from build123d import *

# Parameters (mm, degrees)
SKETCH1_W           = 200
SKETCH1_H           = 120
BOSS_EXTRUDE3_DEPTH = 10
SKETCH3_R           = 5
SKETCH3_W           = 160
SKETCH3_H           = 80
CUT_EXTRUDE2_DEPTH  = 5
SKETCH6_R           = 9
SKETCH6_R_2         = 5.25
BOSS_EXTRUDE4_DEPTH = 10
CHAMFER1_SIZE       = 1


with BuildPart() as part:
    # Sketch1 → Boss-Extrude3 (new body)
    with BuildSketch(Plane(origin=(0, 0, 0), x_dir=(1, 0, 0), z_dir=(0, 1, 0))):
        Rectangle(SKETCH1_W, SKETCH1_H)
    extrude(amount=BOSS_EXTRUDE3_DEPTH)

    # Sketch3 → Cut-Extrude2 (cut)
    with BuildSketch(Plane(origin=(0, 10, 0), x_dir=(1, 0, 0), z_dir=(0, 1, 0))):
        with Locations(Location((-90, 50, 0), (0, 0, 270))):
            Circle(SKETCH3_R)
        with Locations(Location((90, -50, 0), (0, 0, 270))):
            Circle(SKETCH3_R)
        with Locations(Location((90, 50, 0), (0, 0, 270))):
            Circle(SKETCH3_R)
        with Locations(Location((-90, -50, 0), (0, 0, 270))):
            Circle(SKETCH3_R)
        Rectangle(SKETCH3_W, SKETCH3_H)
    extrude(amount=-CUT_EXTRUDE2_DEPTH, mode=Mode.SUBTRACT)

    # Sketch6 → Boss-Extrude4 (add)
    # profile 1 of 4: a face of its own
    with BuildSketch(Plane(origin=(0, 5, 0), x_dir=(1, 0, 0), z_dir=(0, 1, 0))):
        with Locations(Location((-90, 50, 0), (0, 0, 270))):
            Circle(SKETCH6_R)
        with Locations(Location((-90, 50, 0), (0, 0, 270))):
            Circle(SKETCH6_R_2, mode=Mode.SUBTRACT)
    # profile 2 of 4: a face of its own
    with BuildSketch(Plane(origin=(0, 5, 0), x_dir=(1, 0, 0), z_dir=(0, 1, 0))):
        with Locations(Location((90, 50, 0), (0, 0, 270))):
            Circle(SKETCH6_R)
        with Locations(Location((90, 50, 0), (0, 0, 270))):
            Circle(SKETCH6_R_2, mode=Mode.SUBTRACT)
    # profile 3 of 4: a face of its own
    with BuildSketch(Plane(origin=(0, 5, 0), x_dir=(1, 0, 0), z_dir=(0, 1, 0))):
        with Locations(Location((90, -50, 0), (0, 0, 270))):
            Circle(SKETCH6_R)
        with Locations(Location((90, -50, 0), (0, 0, 270))):
            Circle(SKETCH6_R_2, mode=Mode.SUBTRACT)
    # profile 4 of 4: a face of its own
    with BuildSketch(Plane(origin=(0, 5, 0), x_dir=(1, 0, 0), z_dir=(0, 1, 0))):
        with Locations(Location((-90, -50, 0), (0, 0, 270))):
            Circle(SKETCH6_R)
        with Locations(Location((-90, -50, 0), (0, 0, 270))):
            Circle(SKETCH6_R_2, mode=Mode.SUBTRACT)
    extrude(amount=BOSS_EXTRUDE4_DEPTH)

    # Chamfer1
    chamfer1_edges = [part.edges().sort_by_distance(p)[0] for p in [
        (-90, 10, -59),
        (90, 10, -59),
        (90, 10, 41),
        (-90, 10, 41),
    ]]
    chamfer(chamfer1_edges, length=CHAMFER1_SIZE - 0.0001)  # a hair under: the kernel refuses the full size


solid = part.part
Work out the finished part from the listing and answer in its coordinate system (mm). A direction names the side the tool comes from. Coordinates: 2 decimals unless noted, no trailing zeros. Write each loop counter-clockwise with the first axis right and the second up, starting at its lowest first coordinate (ties: lowest second). Pieces come first, ordered by that corner, then holes. Notation, with made-up numbers: M -13,64 L 14,64 A26 ccw 14,96 Z; hole C 82,59.25 d11. An arc over 180 degrees is marked long. Answer as CSV lines item,"result". Start each with the question number.
Item 1: Consider L1, parallel to X at y = 12.4, z = -50; L2, parallel to X at y = 7.75, z = 15; L3, parallel to Z at x = 35.5, y = 6. Determine where each line is inside the solid, lowest interval first.
Item 2: A tool of negligible diameter and unlimited length cuts with its end or side. For faces 1 (the face through (-1, 0, -1)), 2 (the face through (-1, 10, -41)), from which of +Z, -Z, +X, -X, +Y, -Y can it reach the whole face along a straight path? Write none if from no direction.
Item 3: Section A-A on x = -48.5 is taken. Write down the section's boundary in (y, z).
Item 4: Section C-C on z = -10.5 is taken. Write down the section's boundary in (x, y).
Item 5: Determine the mould class of faces 3 (the face through (-94.88, 7.54, 48.92)), 4 (the face through (86, 15, 54)), 5 (the face through (-1, 5, -1)), 6 (the face through (-1, 5, -60)) for opening direction Z: released by +Z, released by -Z, zero draft, split by the parting line, or undercut.
Item 6: A flat-ended cylindrical pin translates along its axis: P1, Ø4, axis at x = -50, z = 11.5, coming from the +Y side. Find the tip coordinate at first contact, or state that the pin passes through.
Checks:
1,L1,"x = -99 to -95.25, -84.75 to -81, 81 to 84.75, 95.25 to 99"
1,L2,"x = -100 to -80, 80 to 100"
1,L3,"z = -60 to -40, 40 to 60"
2,face 1,"+Z, -Z, +X, -X, -Y"
2,face 2,"+Y"
3,outline,"M 0,-60 L 10,-60 L 10,-40 L 5,-40 L 5,40 L 10,40 L 10,60 L 0,60 Z"
4,outline,"M -100,0 L 100,0 L 100,10 L 80,10 L 80,5 L -80,5 L -80,10 L -100,10 Z"
5,face 3,"undercut"
5,face 4,"zero draft"
5,face 5,"undercut"
5,face 6,"released by -Z"
6,P1,"stops at y = 5"
